Design review of the part built by this model. Coordinates are the model's own, in mm. A direction names the side the tool comes from. Give positions to 0.01 mm unless a question says otherwise; leave off trailing zeros. Loops run counter-clockwise (first coordinate to the right, second up) from the corner with the lowest first, then second, coordinate; pieces in that order, holes last. Notation, with made-up numbers: (5, 29.5) -> (18, 29.5) arc R15 ccw to (18, 34.5) -> close; hole circle Ø9 at (27, -6.75). An arc over 180 degrees is marked (long way). Answer as CSV lines item,"result".
from build123d import *

# Parameters (mm, degrees)
BOSS_EXTRUDE1_DEPTH            = 6.35
F_1_4_0_2500_DOWEL_HOLE1_D     = 6.35
F_1_4_0_2500_DOWEL_HOLE1_DEPTH = 6.35
FILLET1_R                      = 6.35
FILLET2_R                      = 1.5875


with BuildPart() as part:
    # Sketch1 → Boss-Extrude1 (new body)
    with BuildSketch(Plane.XY):
        with BuildLine():
            Line((-26.9875, 50.8), (-26.9875, 152.4))
            Line((-26.9875, 152.4), (-50.8, 152.4))
            Line((-50.8, 152.4), (-50.8, -152.4))
            Line((-50.8, -152.4), (-26.9875, -152.4))
            Line((-26.9875, -152.4), (-26.9875, -127))
            ThreePointArc((-26.9875, -127), (0, -100.0125), (26.9875, -127))
            Line((26.9875, -127), (26.9875, -152.4))
            Line((26.9875, -152.4), (50.8, -152.4))
            Line((50.8, -152.4), (50.8, 152.4))
            Line((50.8, 152.4), (26.9875, 152.4))
            Line((26.9875, 152.4), (26.9875, 50.8))
            ThreePointArc((26.9875, 50.8), (0, 23.8125), (-26.9875, 50.8))
        make_face()
    extrude(amount=BOSS_EXTRUDE1_DEPTH)

    # 1/4 (0.2500) Dowel Hole1
    with Locations(Plane.XY.offset(6.35)):
        with Locations((-38.89375, 95.25), (38.89375, 95.25), (38.89375, -95.25), (-38.89375, -95.25)):
            Hole(F_1_4_0_2500_DOWEL_HOLE1_D / 2, depth=F_1_4_0_2500_DOWEL_HOLE1_DEPTH)

    # Fillet1
    fillet1_edges = [part.edges().sort_by_distance(p)[0] for p in [
        (26.9875, -152.4, 3.175),
        (-26.9875, -152.4, 3.175),
        (-26.9875, 152.4, 3.175),
        (26.9875, 152.4, 3.175),
    ]]
    fillet(fillet1_edges, radius=FILLET1_R)

    # Fillet2
    fillet2_edges = [part.edges().sort_by_distance(p)[0] for p in [
        (-50.8, -152.4, 3.175),
        (-50.8, 152.4, 3.175),
        (50.8, 152.4, 3.175),
        (50.8, -152.4, 3.175),
    ]]
    fillet(fillet2_edges, radius=FILLET2_R)


solid = part.part
Q1. We need section D-D, the plane y = 46. State the section outline as (x, z) points, and give its area (3 significant figures).
Filled sheet:
outline,"(-50.8, 0) -> (-26.56, 0) -> (-26.56, 6.35) -> (-50.8, 6.35) -> close; (26.56, 0) -> (50.8, 0) -> (50.8, 6.35) -> (26.56, 6.35) -> close"
area,"308 mm^2"
Q2. The part is to be moulded in two halves that separate along X. For faces 4 (the flat face through (-1, -32, 6.35)), 5 (the cylindrical face through (-28.9, -150.59, 3.22)), 6 (the flat face through (50.8, -2, 3)), say which applies: pulls with the +X half, pulls with the -X half, needs draft (parallel to the pull), parting line crosses it, or undercut.
Filled sheet:
face 4,"needs draft"
face 5,"undercut"
face 6,"pulls with the +X half"
Q3. We need section A-A, the plane y = 95.25. State the section outline as (x, z) points, and give its area (3 significant figures).
Filled sheet:
outline,"(-50.8, 0) -> (-42.07, 0) -> (-42.07, 6.35) -> (-50.8, 6.35) -> close; (-35.72, 0) -> (-26.99, 0) -> (-26.99, 6.35) -> (-35.72, 6.35) -> close; (26.99, 0) -> (35.72, 0) -> (35.72, 6.35) -> (26.99, 6.35) -> close; (42.07, 0) -> (50.8, 0) -> (50.8, 6.35) -> (42.07, 6.35) -> close"
area,"222 mm^2"
Q4. We need section C-C, the plane y = -95.25. State the section outline as (x, z) points.
Filled sheet:
outline,"(-50.8, 0) -> (-42.07, 0) -> (-42.07, 6.35) -> (-50.8, 6.35) -> close; (-35.72, 0) -> (35.72, 0) -> (35.72, 6.35) -> (-35.72, 6.35) -> close; (42.07, 0) -> (50.8, 0) -> (50.8, 6.35) -> (42.07, 6.35) -> close"
Q5. We need section B-B, the plane z = 3. State how many separate pieces and enclosed holes the cut face has, and give its area (3 significant figures).
Filled sheet:
separate pieces,"1"
enclosed holes,"4"
area,"21,700 mm^2"
Q6. For faces 1 (the flat face through (-26.988, -137, 3)), 2 (the flat face through (-41, -152.4, 3)), 3 (the flat face through (26.988, 99, 3)), list the 3-axis set-ups (+Z, -Z, +X, -X, +Y, -Y) from which the entire face can be reached by the end or side of a thin tool; tool diameter is ignored.
Filled sheet:
face 1,"+Z, -Z, -Y"
face 2,"+Z, -Z, +X, -X, -Y"
face 3,"+Z, -Z, +Y"
Q7. To check wall thickness, follow probe 1 along X at (y, z) = (95.5, 0.5); probe 2 along X at (y, z) = (-130.5, 1.25); probe 3 along Y at (x, z) = (36, 5.75). State the ranges of each line that lie inside material, in increasing order. Write a range as from..to.
Filled sheet:
probe 1,"x = -50.8..-42.06, -35.73..-26.99, 26.99..35.73, 42.06..50.8"
probe 2,"x = -50.8..-26.99, 26.99..50.8"
probe 3,"y = -152.4..-96.56, -93.94..93.94, 96.56..152.4"
Q8. Clearance check with flat-ended pins moving along their axes: pin 1 Ø5 at (x, y) = (-18.5, -94) entering from -Z; pin 2 Ø5.5 at (x, y) = (38.89, 95.25) entering from -Z (3 decimals); pin 3 Ø1.5 at (x, z) = (1, 4.5) entering from -Y. State where each tip first meets the part, or that it passes through.
Filled sheet:
pin 1,"stops at z = 0"
pin 2,"passes through"
pin 3,"stops at y = -100.07"
